For this review, take the finished solid that the model builds, in its own axes (mm). A direction names the side the tool comes from. Coordinates: 2 decimals unless noted, no trailing zeros. Loops run counter-clockwise (first coordinate to the right, second up) from the corner with the lowest first, then second, coordinate; pieces in that order, holes last. Notation, with made-up numbers: (54, -24.75) - (105, -24.75) arc R22 ccw to (105, 2.25) - close; hole circle Ø7 at (50.5, 30.25). An arc over 180 degrees is marked (long way). One line per item, written item: value. Start each with the question number.
1. Take a section at D-D, the plane z = 2.15. State the section outline as (x, y) points.
2. Insertion check: pin 1 (1.5 mm diameter, centred on x = 1, y = -3, fed in from +Z); pin 2 (1.5 mm diameter, centred on y = -3.5, z = -1, fed in from -X); pin 3 (2 mm diameter, centred on y = 1, z = 1.5, fed in from +X). Each pin has a flat end and moves straight along its axis. Give the tip position at first contact, or say it passes through.
3. For faces 1 (the face through (0, 0, -2)), 2 (the face through (-0.1, -3.2, 0)), list the 3-axis set-ups (+Z, -Z, +X, -X, +Y, -Y) from which the entire face can be reached by the end or side of a thin tool; tool diameter is ignored.
4. Take a section at A-A, the plane y = 0. State the section outline as (x, z) points.
5. Take a section at C-C, the plane z = -0.3. State the section outline as (x, y) points.
6. To check wall thickness, follow line 1 (Z direction, x = 3, y = -0.5); line 2 (X direction, y = 1.5, z = 1.7); line 3 (X direction, y = 1, z = -1.3). State the ranges of each line that lie inside material, in increasing order. Write a range as from..to.
```python
from build123d import *

# Parameters (mm, degrees)
SKETCH_R        = 4.9
PAD_DEPTH       = 2
SKETCH001_R     = 2
PAD001_DEPTH    = 3
CHAMFER_SIZE    = 1
CHAMFER001_SIZE = 0.6


with BuildPart() as part:
    # Sketch → Pad (new body)
    with BuildSketch(Plane.XY):
        Circle(SKETCH_R)
    extrude(amount=-PAD_DEPTH)

    # Sketch001 → Pad001 (join)
    with BuildSketch(Plane.XY):
        Circle(SKETCH001_R)
    extrude(amount=PAD001_DEPTH)

    # Chamfer
    chamfer_edges = [part.edges().sort_by_distance(p)[0] for p in [
        (-2, 0, 0),
    ]]
    chamfer(chamfer_edges, length=CHAMFER_SIZE)

    # Chamfer001
    chamfer001_edges = [part.edges().sort_by_distance(p)[0] for p in [
        (-4.9, 0, -2),
    ]]
    chamfer(chamfer001_edges, length=CHAMFER001_SIZE)


solid = part.part
```
Solutions:
1. outline: circle Ø4 at (0, 0)
2. pin 1: z = 0.59
2. pin 2: x = -4.06
2. pin 3: x = 2.35
3. face 1: -Z, +X, -X, +Y, -Y
3. face 2: +Z
4. outline: (-4.9, -1.4) - (-4.3, -2) - (4.3, -2) - (4.9, -1.4) - (4.9, 0) - (3, 0) - (2, 1) - (2, 3) - (-2, 3) - (-2, 1) - (-3, 0) - (-4.9, 0) - close
5. outline: circle Ø9.8 at (0, 0)
6. line 1: -2..0
6. line 2: -1.32..1.32
6. line 3: -4.8..4.8
